For this review, take the finished solid that the model builds, in its own axes (mm). Face numbers are marked on the shaded views. Give positions to 0.01 mm unless a question says otherwise; leave off trailing zeros. Order: outer loops, then holes, each group sorted by start corner. A loop starts at its lowest first (then second) coordinate and runs counter-clockwise, first axis right, second up. Notation, with made-up numbers: (40, 1) - (81, 1) arc R21 cw to (81, 30) - close; hole circle Ø2 at (22, -32). An arc over 180 degrees is marked (long way). One line per item, written item: value.
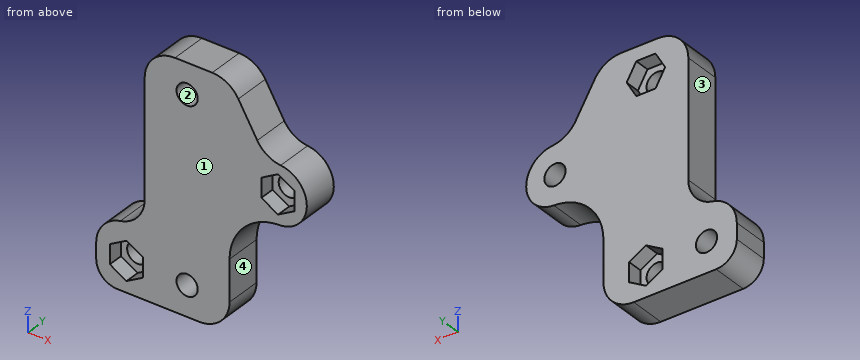
```python
from build123d import *

# Parameters (mm, degrees)
SKETCH2_W           = 35
SKETCH2_H           = 40
SKETCH2_R           = 1.75
BOSS_EXTRUDE2_DEPTH = 6
CUT_EXTRUDE1_DEPTH  = 2.5
CUT_EXTRUDE2_DEPTH  = 2.5
CUT_EXTRUDE3_DEPTH  = 7
FILLET3_R           = 5
FILLET4_R           = 8.5


with BuildPart() as part:
    # Sketch2 → Boss-Extrude2 (new body)
    with BuildSketch(Plane(origin=(0, 0, 0), x_dir=(1, 0, 0), z_dir=(0, 1, 0))):
        with Locations((17.5, 20)):
            Rectangle(SKETCH2_W, SKETCH2_H)
        with Locations((5, 35)):
            Circle(SKETCH2_R, mode=Mode.SUBTRACT)
        with Locations((30, 15)):
            Circle(SKETCH2_R, mode=Mode.SUBTRACT)
        with Locations((15, 35)):
            Circle(SKETCH2_R, mode=Mode.SUBTRACT)
        with Locations((15, 5)):
            Circle(SKETCH2_R, mode=Mode.SUBTRACT)
    extrude(amount=BOSS_EXTRUDE2_DEPTH)

    # Sketch3 → Cut-Extrude1 (cut)
    with BuildSketch(Plane.XZ):
        Polygon((7.75, -36.58771324), (7.75, -33.41228676), (5, -31.824573519), (2.25, -33.41228676), (2.25, -36.58771324), (5, -38.175426481), align=None)
        Polygon((30, -11.824573519), (27.25, -13.41228676), (27.25, -16.58771324), (30, -18.175426481), (32.75, -16.58771324), (32.75, -13.41228676), align=None)
    extrude(amount=-CUT_EXTRUDE1_DEPTH, mode=Mode.SUBTRACT)

    # Sketch4 → Cut-Extrude2 (cut)
    with BuildSketch(Plane(origin=(0, 6, 0), x_dir=(1, 0, 0), z_dir=(0, 1, 0))):
        Polygon((17.75, 36.58771324), (15, 38.175426481), (12.25, 36.58771324), (12.25, 33.41228676), (15, 31.824573519), (17.75, 33.41228676), align=None)
        Polygon((13.41228676, 7.75), (11.824573519, 5), (13.41228676, 2.25), (16.58771324, 2.25), (18.175426481, 5), (16.58771324, 7.75), align=None)
    extrude(amount=-CUT_EXTRUDE2_DEPTH, mode=Mode.SUBTRACT)

    # Sketch5 → Cut-Extrude3 (cut, through all)
    with BuildSketch(Plane(origin=(0, 6, 0), x_dir=(1, 0, 0), z_dir=(0, 1, 0))):
        with BuildLine():
            Line((0, 36.58771324), (0, 40))
            Line((0, 40), (3.41228676, 40))
            ThreePointArc((3.41228676, 40), (0.999435653, 39.000564347), (0, 36.58771324))
        make_face()
        with BuildLine():
            Line((30, 19.75), (22, 19.75))
            Line((22, 19.75), (22, 40))
            Line((22, 40), (35, 40))
            Line((35, 40), (35, 0))
            Line((35, 0), (22, 0))
            Line((22, 0), (28, 10.25))
            Line((28, 10.25), (30, 10.25))
            ThreePointArc((30, 10.25), (34.75, 15), (30, 19.75))
        make_face()
        with BuildLine():
            Line((0, 34), (0, 0))
            Line((0, 0), (8, 0))
            Line((8, 0), (8, 29))
            Line((8, 29), (5, 29))
            ThreePointArc((5, 29), (1.464466094, 30.464466094), (0, 34))
        make_face()
    extrude(amount=-CUT_EXTRUDE3_DEPTH, mode=Mode.SUBTRACT)

    # Fillet3
    fillet3_edges = [part.edges().sort_by_distance(p)[0] for p in [
        (28, 3, -10.25),
        (22, 3, 0),
        (22, 3, -40),
        (8, 3, -29),
        (8, 3, 0),
    ]]
    fillet(fillet3_edges, radius=FILLET3_R)

    # Fillet4
    fillet4_edges = [part.edges().sort_by_distance(p)[0] for p in [
        (22, 3, -19.75),
    ]]
    fillet(fillet4_edges, radius=FILLET4_R)


solid = part.part
```
(1) Wall thickness on line 1 (X direction, y = 4.9, z = -35); line 2 (Z direction, x = 15, y = 0.9); line 3 (X direction, y = 2.35, z = -35): over which ranges is each line inside the solid? List them lowest first. Write a range as from..to.
Answers below:
line 1: x = 0..3.25, 6.75..12.25, 17.75..22
line 2: z = -40..-36.75, -33.25..-6.75, -3.25..0
line 3: x = 0..2.25, 7.75..13.25, 16.75..22
(2) Take a section at C-C (x = 8.5). Write out the cut boundary in (y, z).
Answers below:
outline: (0, -40) - (6, -40) - (6, -2.82) - (0, -2.82) - close
(3) Take a section at B-B (y = 0.5). Give the number of separate pieces and of enclosed holes in the cut face, then the cut area to 3 significant figures.
Answers below:
separate pieces: 1
enclosed holes: 4
area: 720 mm^2
(4) Take a section at A-A (z = -15). Write out the cut boundary in (x, y), then the cut area to 4 significant figures.
Answers below:
outline: (8, 0) - (27.25, 0) - (27.25, 2.5) - (28.25, 2.5) - (28.25, 6) - (8, 6) - close; (31.75, 2.5) - (32.75, 2.5) - (32.75, 0) - (34.75, 0) - (34.75, 6) - (31.75, 6) - close
area: 134.5 mm^2
(5) For P1, Ø0.8, axis at y = 1, z = -15, coming from the -X side; P2, Ø1, axis at x = 12, z = -8.5, coming from the -Y side; P3, Ø2, axis at x = 15, z = -5, coming from the -Y side; P4, Ø2, axis at y = 5, z = -35, coming from the +X side, all flat-tipped, find the tip position at first contact; note any pin that passes through.
Answers below:
P1: stops at x = 8
P2: stops at y = 0
P3: passes through
P4: stops at x = 22
(6) Draft analysis for pull direction X (two halves, no side actions). For the marked faces 1, 2, 3 and 4, state which applies: pulls with the +X half, pulls with the -X half, needs draft (parallel to the pull), parting line crosses it, or undercut.
Answers below:
face 1: needs draft
face 2: undercut
face 3: pulls with the -X half
face 4: pulls with the +X half
